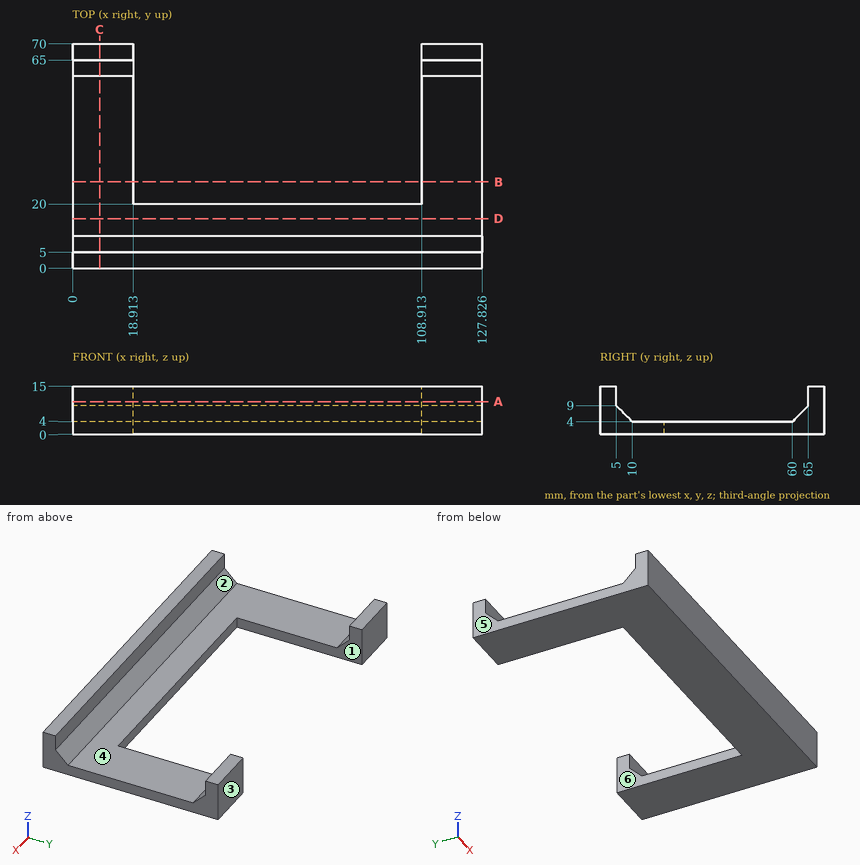
Source: three-view drawing plus pictorial views. Frame: mm from the lowest corner of the part. A direction names the side the tool comes from. Coordinates: 2 decimals unless noted, no trailing zeros. Loops run counter-clockwise (first coordinate to the right, second up) from the corner with the lowest first, then second, coordinate; pieces in that order, holes last. Notation, with made-up numbers: (-34.5, 14.25) -> (-16.5, 14.25) arc R22 ccw to (-16.5, 43.25) -> close; hole circle Ø2 at (50.25, 14.25). An arc over 180 degrees is marked (long way). Answer in a Markdown table with one row per item. Add a question column.
Q1. Pull-direction query (Y, two-part tool) for the marked faces 1, 2 and 3; classes: pulls with the +Y half, pulls with the -Y half, needs draft (parallel to the pull), parting line crosses it, or undercut.
Q2. Section C-C on x = 8.5. Return the cut outline in (y, z).
Q3. Ray query, line 1 along X through (y, z) = (34, 3); line 2 along Y through (x, z) = (20.5, 11.25); line 3 along Y through (x, z) = (15.5, 8.5). Return the intervals inside material, ascending.
Q4. Contact query for flat-ended pins moving along their axis: pin 1 Ø1 at (x, z) = (93.5, 5.5) entering from -Y; pin 2 Ø1.2 at (x, z) = (53.5, 2) entering from +Y; pin 3 Ø5 at (x, z) = (61.5, 11) entering from +Y. Output: stop coordinate, or through.
Q5. Section A-A on z = 10.25. Return the cut outline in (x, y), and give its area (3 significant figures).
Q6. Section B-B on y = 27. Return the cut outline in (x, z).
Q7. Reachability of the marked faces 4, 5 and 6 from +Z, -Z, +X, -X, +Y, -Y: full face, straight path, thin tool, end or side. Return the list, or none.
Q8. Section D-D on y = 15.5. Return the cut outline in (x, z), and give its area (3 significant figures).
Computed values:
| question | item | result |
|---|---|---|
| 1 | face 1 | needs draft |
| 1 | face 2 | undercut |
| 1 | face 3 | pulls with the +Y half |
| 2 | outline | (0, 0) -> (70, 0) -> (70, 15) -> (65, 15) -> (65, 9) -> (60, 4) -> (10, 4) -> (5, 9) -> (5, 15) -> (0, 15) -> close |
| 3 | line 1 | x = 0 to 18.91, 108.91 to 127.83 |
| 3 | line 2 | y = 0 to 5 |
| 3 | line 3 | y = 0 to 5.5, 64.5 to 70 |
| 4 | pin 1 | stops at y = 0 |
| 4 | pin 2 | stops at y = 20 |
| 4 | pin 3 | stops at y = 5.5 |
| 5 | outline | (0, 0) -> (127.83, 0) -> (127.83, 5) -> (0, 5) -> close; (0, 65) -> (18.91, 65) -> (18.91, 70) -> (0, 70) -> close; (108.91, 65) -> (127.83, 65) -> (127.83, 70) -> (108.91, 70) -> close |
| 5 | area | 828 mm^2 |
| 6 | outline | (0, 0) -> (18.91, 0) -> (18.91, 4) -> (0, 4) -> close; (108.91, 0) -> (127.83, 0) -> (127.83, 4) -> (108.91, 4) -> close |
| 7 | face 4 | +Z, +X, -X |
| 7 | face 5 | +Z, -Z, -X, +Y, -Y |
| 7 | face 6 | +Z, -Z, +Y |
| 8 | outline | (0, 0) -> (127.83, 0) -> (127.83, 4) -> (0, 4) -> close |
| 8 | area | 511 mm^2 |
